from build123d import *

# Parameters (mm, degrees)
F0_W     = 35.56
F0_H     = 38.1
F1_DEPTH = 25.4
F2_T     = -2.54
F3_W     = 25.4
F3_H     = 20.575015
F4_DEPTH = 25.4


with BuildPart() as f1:
    # F0 (on Top) → F1 (new body)
    with BuildSketch(Plane.XY):
        Rectangle(F0_W, F0_H)
    extrude(amount=F1_DEPTH)

    # F2
    f2_openings = [f1.faces().sort_by_distance(p)[0] for p in [
        (0, 0, 25.4),
    ]]
    offset(amount=F2_T, openings=f2_openings)

    # F3 (on Top) → F4 (cut)
    with BuildSketch(Plane.XY):
        with Locations((27.727038, -1.20786)):
            Rectangle(F3_W, F3_H)
    extrude(amount=F4_DEPTH, mode=Mode.SUBTRACT)


solid = f1.part
The listing builds one solid part. Answer for the finished solid, in the listing's coordinates (mm). A direction names the side the tool comes from. Give positions to 0.01 mm unless a question says otherwise; leave off trailing zeros. Loops run counter-clockwise (first coordinate to the right, second up) from the corner with the lowest first, then second, coordinate; pieces in that order, holes last.
Item 1: Find the intervals of material crossed by line 1 along Y through (x, z) = (-12.5, 3.25); line 2 along Y through (x, z) = (16.5, 16.75); line 3 along X through (y, z) = (-13, 23.5), in increasing order.
Derived:
line 1: y = -19.05 to -16.51, 16.51 to 19.05
line 2: y = -19.05 to -11.5, 9.08 to 19.05
line 3: x = -17.78 to -15.24, 15.24 to 17.78
Item 2: A tool of negligible diameter and unlimited length cuts with its end or side. For faces 4 (the flat face through (-16, 2, 25.4)), 5 (the flat face through (15.24, -14, 14)), 6 (the flat face through (16, -11.495, 13)), from which of +Z, -Z, +X, -X, +Y, -Y can it reach the whole face along a straight path? Write none if from no direction.
Derived:
face 4: +Z, +X, -X, +Y, -Y
face 5: +Z
face 6: +Z, -Z, +X
Item 3: Determine the mould class of faces 1 (the flat face through (0, 0, 2.54)), 2 (the flat face through (-17.78, 0, 13)), 3 (the flat face through (0, -19.05, 13)) for opening direction Y: +Y half, -Y half, draft (parallel to the pull), parting line (faces both ways), or undercut.
Derived:
face 1: undercut
face 2: draft
face 3: -Y half
Item 4: Each of these flat-tipped pins is pushed along its axis until it touches: pin 1 Ø10 at (x, y) = (-4.5, 15) entering from +Z; pin 2 Ø6 at (y, z) = (-7, 16) entering from +X; pin 3 Ø9 at (x, y) = (5, 0.5) entering from +Z; pin 4 Ø2 at (y, z) = (1.5, 1) entering from +X. Where does it stop, or does it pass through?
Derived:
pin 1: stops at z = 25.4
pin 2: stops at x = -15.24
pin 3: stops at z = 2.54
pin 4: stops at x = 15.03
Item 5: A cutting plane is placed at D-D (x = 4.5). Give the vertices of the cut face in (y, z).
Derived:
outline: (-19.05, 0) - (19.05, 0) - (19.05, 25.4) - (16.51, 25.4) - (16.51, 2.54) - (-16.51, 2.54) - (-16.51, 25.4) - (-19.05, 25.4) - close
Item 6: A cutting plane is placed at A-A (x = 16.5). Give the vertices of the cut face in (y, z).
Derived:
outline: (-19.05, 0) - (-11.5, 0) - (-11.5, 25.4) - (-19.05, 25.4) - close; (9.08, 0) - (19.05, 0) - (19.05, 25.4) - (9.08, 25.4) - close
Item 7: A cutting plane is placed at C-C (y = 3). Give the vertices of the cut face in (x, z).
Derived:
outline: (-17.78, 0) - (15.03, 0) - (15.03, 2.54) - (-15.24, 2.54) - (-15.24, 25.4) - (-17.78, 25.4) - close
Item 8: A cutting plane is placed at B-B (z = 17). Give the vertices of the cut face in (x, y).
Derived:
outline: (-17.78, -19.05) - (17.78, -19.05) - (17.78, -11.5) - (15.24, -11.5) - (15.24, -16.51) - (-15.24, -16.51) - (-15.24, 16.51) - (15.24, 16.51) - (15.24, 9.08) - (17.78, 9.08) - (17.78, 19.05) - (-17.78, 19.05) - close
